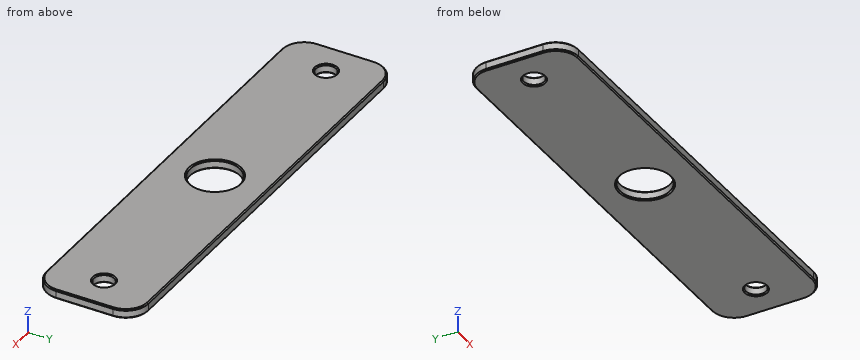
from build123d import *

# Parameters (mm, degrees)
ESQUISSE1_W        = 200
ESQUISSE1_H        = 45
BOSS_EXTRU_1_DEPTH = 4
CONG_2_R           = 10
D_GAGEMENT_M81_D   = 9
D_GAGEMENT_M201_D  = 22
CHANFREIN2_SIZE    = 0.5
CHANFREIN3_SIZE    = 0.5


with BuildPart() as part:
    # Esquisse1 → Boss.-Extru.1 (new body)
    with BuildSketch(Plane.XY):
        with Locations((-21.919003271, 59.078947368)):
            Rectangle(ESQUISSE1_W, ESQUISSE1_H)
    extrude(amount=BOSS_EXTRU_1_DEPTH)

    # Congé2
    cong_2_edges = [part.edges().sort_by_distance(p)[0] for p in [
        (-121.919003271, 81.578947368, 2),
        (78.080996729, 81.578947368, 2),
        (78.080996729, 36.578947368, 2),
        (-121.919003271, 36.578947368, 2),
    ]]
    fillet(cong_2_edges, radius=CONG_2_R)

    # Dégagement M81 (through all)
    with Locations(Plane.XY.offset(4)):
        with Locations((-106.919003271, 59.078947368), (63.080996729, 59.078947368)):
            Hole(D_GAGEMENT_M81_D / 2)

    # Dégagement M201 (through all)
    with Locations(Plane.XY.offset(4)):
        with Locations((-21.919003271, 59.078947368)):
            Hole(D_GAGEMENT_M201_D / 2)

    # Chanfrein2
    chanfrein2_edges = [part.edges().sort_by_distance(p)[0] for p in [
        (-121.919003271, 59.078947368, 0),
        (-121.919003271, 59.078947368, 4),
        (-21.919003271, 81.578947368, 0),
        (78.080996729, 59.078947368, 0),
        (-21.919003271, 36.578947368, 0),
        (75.15206454, 78.65001518, 0),
        (75.15206454, 39.507879557, 0),
        (-118.990071083, 39.507879557, 0),
        (-118.990071083, 78.65001518, 0),
        (-21.919003271, 81.578947368, 4),
        (-21.919003271, 36.578947368, 4),
        (78.080996729, 59.078947368, 4),
        (75.15206454, 78.65001518, 4),
        (75.15206454, 39.507879557, 4),
        (-118.990071083, 39.507879557, 4),
        (-118.990071083, 78.65001518, 4),
    ]]
    chamfer(chanfrein2_edges, length=CHANFREIN2_SIZE)

    # Chanfrein3
    chanfrein3_edges = [part.edges().sort_by_distance(p)[0] for p in [
        (67.580996729, 59.078947368, 4),
        (67.580996729, 59.078947368, 0),
        (-102.419003271, 59.078947368, 4),
        (-102.419003271, 59.078947368, 0),
        (-10.919003271, 59.078947368, 4),
        (-10.919003271, 59.078947368, 0),
    ]]
    chamfer(chanfrein3_edges, length=CHANFREIN3_SIZE)


solid = part.part
Input: part model. Units: mm. Frame: model coordinates. Give positions to 0.01 mm unless a question says otherwise; leave off trailing zeros. Write each loop counter-clockwise with the first axis right and the second up, starting at its lowest first coordinate (ties: lowest second). Pieces come first, ordered by that corner, then holes. Notation, with made-up numbers: (-25, 72) -> (16, 72) arc R31 ccw to (16, 109) -> close; hole circle Ø2 at (20.5, -21). An arc over 180 degrees is marked (long way). Use one line per item in the form item = value. Start each with the question number.
1) Ray query, probe 1 along X at (y, z) = (59.5, 3.5); probe 2 along X at (y, z) = (59, 0.4); probe 3 along X at (y, z) = (46, 0.75). Return the intervals inside material, ascending. Write a range as from..to.
2) Section query B-B on y = 56.5. Count the separate pieces of the cut face and the enclosed holes in it, then the cut area to 3 significant figures.
3) Section query A-A on z = 1.35. Return the cut outline in (x, y).
Outcome:
q1.probe_1 = -121.92..-111.4, -102.44..-32.91, -10.93..58.6, 67.56..78.08
q1.probe_2 = -121.82..-111.52, -102.32..-33.02, -10.82..58.48, 67.68..77.98
q1.probe_3 = -121.9..78.06
q2.separate_pieces = 4
q2.enclosed_holes = 0
q2.area = 653 mm^2
q3.outline = (-121.92, 46.58) arc R10 ccw to (-111.92, 36.58) -> (68.08, 36.58) arc R10 ccw to (78.08, 46.58) -> (78.08, 71.58) arc R10 ccw to (68.08, 81.58) -> (-111.92, 81.58) arc R10 ccw to (-121.92, 71.58) -> close; hole circle Ø9 at (-106.92, 59.08); hole circle Ø22 at (-21.92, 59.08); hole circle Ø9 at (63.08, 59.08)
